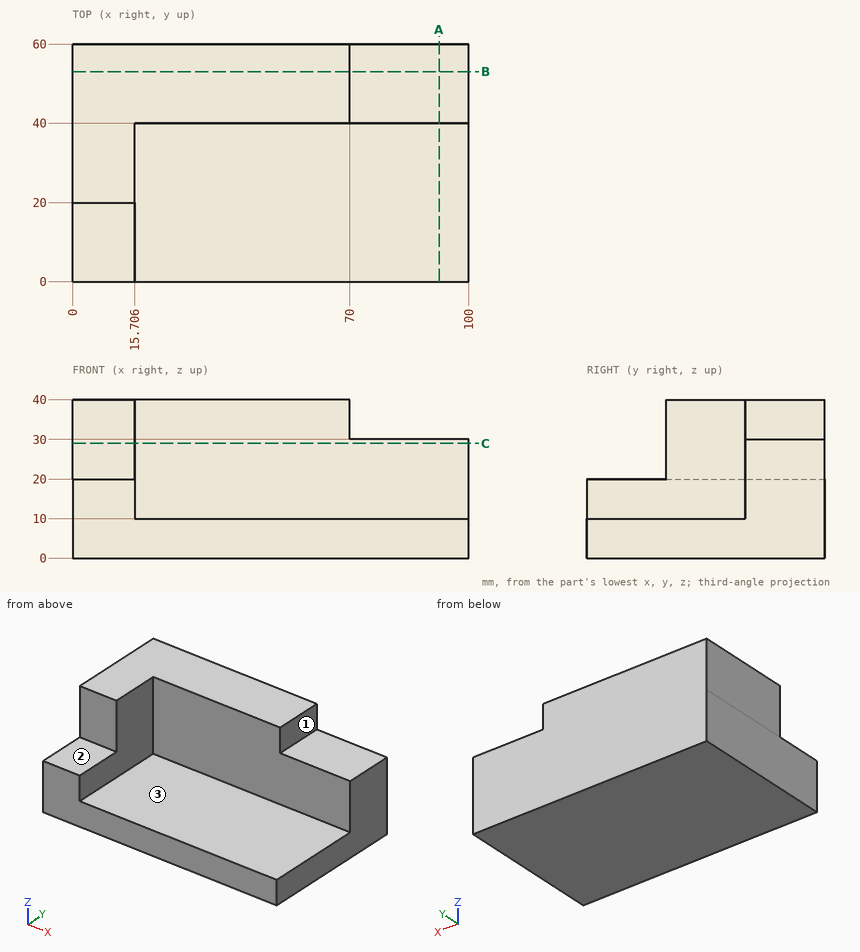
Study the drawing (mm; zero at the part's minimum x, y, z) and answer. A direction names the side the tool comes from. Give positions to 0.01 mm unless a question says otherwise; leave off trailing zeros. Order: outer loops, then holes, each group sorted by start corner. A loop starts at its lowest first (then second) coordinate and runs counter-clockwise, first axis right, second up. Notation, with made-up numbers: (22, -1) - (33, -1) arc R21 ccw to (33, 15) - close; hole circle Ø8 at (-37, 44.25). An arc over 180 degrees is marked (long way). Answer in a Markdown table with one row per item. Add a question column.
Q1. The part is cut by section C-C (z = 29). Determine the outline of the cut face in (x, y), then the cut area to 3 significant figures.
Q2. The part is cut by section B-B (y = 53). Determine the outline of the cut face in (x, z), then the cut area to 3 significant figures.
Q3. Given P1, Ø6, axis at y = 25, z = 13.5, coming from the -X side; P2, Ø20, axis at x = 45.5, y = 17.5, coming from the +Z side; P3, Ø10, axis at x = 86.5, y = 45.5, coming from the +Z side; P4, Ø12.5, axis at x = 5.5, z = 33, coming from the -Y side, each flat-ended and moving along its own axis, determine where each tip first touches the part or whether it passes through.
Q4. Find the intervals of material crossed by line 1 along X through (y, z) = (28, 23.5); line 2 along Y through (x, z) = (65, 32.5); line 3 along Y through (x, z) = (5.5, 28.5), in increasing order. Write a range as [from, to].
Q5. The part is cut by section A-A (x = 92.5). Determine the outline of the cut face in (y, z), then the cut area to 3 significant figures.
Q6. Which of the six approach directions +Z, -Z, +X, -X, +Y, -Y give full straight-line access (tool end or side, diameter ignored) to the marked faces 1, 2 and 3?
Determined:
| question | item | result |
|---|---|---|
| 1 | outline | (0, 20) - (15.71, 20) - (15.71, 40) - (100, 40) - (100, 60) - (0, 60) - close |
| 1 | area | 2,310 mm² |
| 2 | outline | (0, 0) - (100, 0) - (100, 30) - (70, 30) - (70, 40) - (0, 40) - close |
| 2 | area | 3,700 mm² |
| 3 | P1 | stops at x = 0 |
| 3 | P2 | stops at z = 10 |
| 3 | P3 | stops at z = 30 |
| 3 | P4 | stops at y = 20 |
| 4 | line 1 | x = [0, 15.71] |
| 4 | line 2 | y = [40, 60] |
| 4 | line 3 | y = [20, 60] |
| 5 | outline | (0, 0) - (60, 0) - (60, 30) - (40, 30) - (40, 10) - (0, 10) - close |
| 5 | area | 1,000 mm² |
| 6 | face 1 | +Z, +X, +Y, -Y |
| 6 | face 2 | +Z, +X, -X, -Y |
| 6 | face 3 | +Z, +X, -Y |
